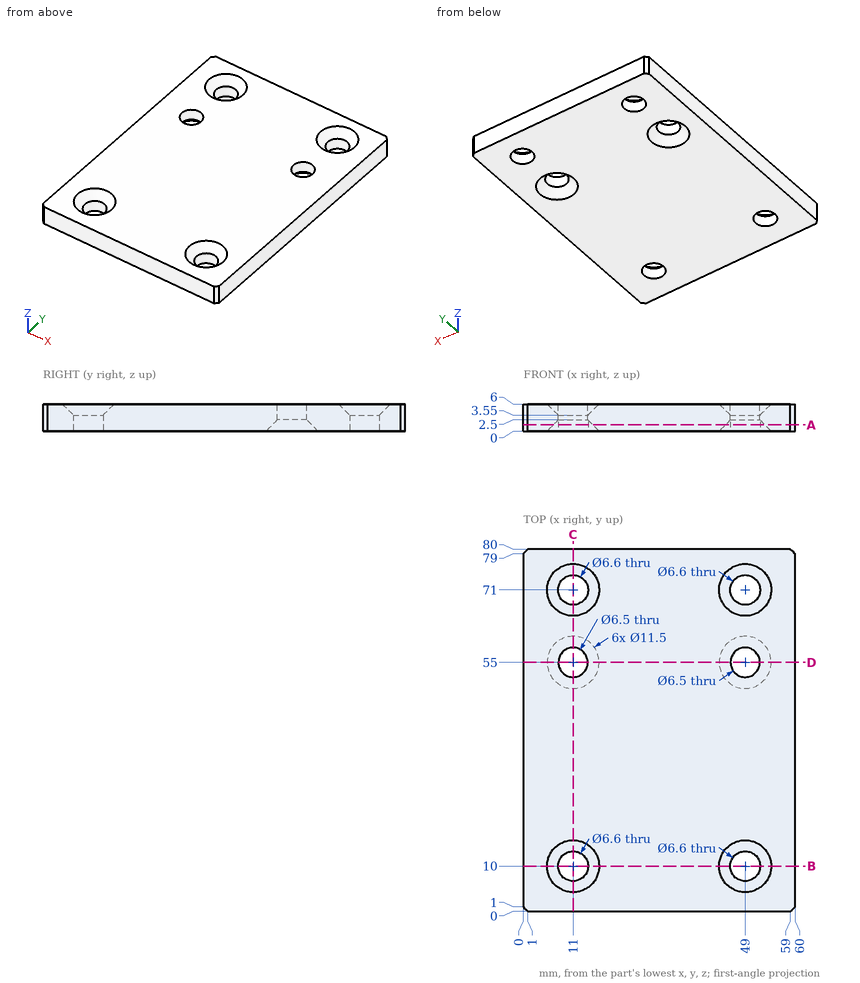
Print and shaded views of the part. All mm, measured from the part's lowest x, y and z. Round coordinates to 2 decimals unless told otherwise and drop trailing zeros. Order: outer loops, then holes, each group sorted by start corner. A loop starts at its lowest first (then second) coordinate and runs counter-clockwise, first axis right, second up.
Q1. Wall check: L1, parallel to X at y = 10, z = 2; L2, parallel to Y at x = 11, z = 2.8; L3, parallel to X at y = 55, z = 5.05. Give the ranges that are in metal, low to high.
Q2. Slice it at A-A (z = 1.4). Write the cut outline in (x, y).
Q3. Drop a flat-ended pin along its axis: pin 1 (4 mm diameter, centred on x = 49, y = 10, fed in from +Z). Give the stop position or say it passes through.
Q4. Slice it at B-B (y = 10). Write the cut outline in (x, z), and give its area (3 significant figures).
Q5. Slice it at D-D (y = 55). Write the cut outline in (x, z).
Q6. Slice it at C-C (x = 11). Write the cut outline in (y, z), and give its area (3 significant figures).
Results below:
1. L1: x = 0 to 7.7, 14.3 to 45.7, 52.3 to 60
1. L2: y = 0 to 6.7, 13.3 to 51.75, 58.25 to 67.7, 74.3 to 80
1. L3: x = 0 to 7.75, 14.25 to 45.75, 52.25 to 60
2. outline: (0, 1) - (1, 0) - (59, 0) - (60, 1) - (60, 79) - (59, 80) - (1, 80) - (0, 79) - close; hole circle Ø8.7 at (11, 55); hole circle Ø6.6 at (11, 10); hole circle Ø6.6 at (11, 71); hole circle Ø8.7 at (49, 55); hole circle Ø6.6 at (49, 10); hole circle Ø6.6 at (49, 71)
3. pin 1: passes through
4. outline: (0, 0) - (7.7, 0) - (7.7, 3.55) - (5.25, 6) - (0, 6) - close; (14.3, 0) - (45.7, 0) - (45.7, 3.55) - (43.25, 6) - (16.75, 6) - (14.3, 3.55) - close; (52.3, 0) - (60, 0) - (60, 6) - (54.75, 6) - (52.3, 3.55) - close
4. area: 269 mm2
5. outline: (0, 0) - (5.25, 0) - (7.75, 2.5) - (7.75, 6) - (0, 6) - close; (14.25, 2.5) - (16.75, 0) - (43.25, 0) - (45.75, 2.5) - (45.75, 6) - (14.25, 6) - close; (52.25, 2.5) - (54.75, 0) - (60, 0) - (60, 6) - (52.25, 6) - close
6. outline: (0, 0) - (6.7, 0) - (6.7, 3.55) - (4.25, 6) - (0, 6) - close; (13.3, 0) - (49.25, 0) - (51.75, 2.5) - (51.75, 6) - (15.75, 6) - (13.3, 3.55) - close; (58.25, 2.5) - (60.75, 0) - (67.7, 0) - (67.7, 3.55) - (65.25, 6) - (58.25, 6) - close; (74.3, 0) - (80, 0) - (80, 6) - (76.75, 6) - (74.3, 3.55) - close
6. area: 344 mm2
